from build123d import *

# Parameters (mm, degrees)
CROQUIS1_R              = 2.5
SALIENTE_EXTRUIR1_DEPTH = 60
CORTAR_EXTRUIR1_START   = -10
CORTAR_EXTRUIR1_DEPTH   = 10
CHAFL_N1_SIZE           = 0.2


with BuildPart() as part:
    # Croquis1 → Saliente-Extruir1 (new body)
    with BuildSketch(Plane(origin=(0, 0, 0), x_dir=(1, 0, 0), z_dir=(0, 1, 0))):
        with Locations(Location((0, 0, 0), (0, 0, 270))):
            Circle(CROQUIS1_R)
    extrude(amount=SALIENTE_EXTRUIR1_DEPTH)

    # Croquis2 → Cortar-Extruir1 (cut)
    with BuildSketch(Plane(origin=(0, 60, 0), x_dir=(1, 0, 0), z_dir=(0, 1, 0)).offset(CORTAR_EXTRUIR1_START)):
        with BuildLine():
            Line((-1.5, 2), (1.5, 2))
            ThreePointArc((1.5, 2), (0, 2.5), (-1.5, 2))
        make_face()
    extrude(amount=CORTAR_EXTRUIR1_DEPTH, mode=Mode.SUBTRACT)

    # Chaflán1
    chafl_n1_edges = [part.edges().sort_by_distance(p)[0] for p in [
        (0, 0, -2.5),
        (-2.371708245, 60, 0.790569415),
    ]]
    chamfer(chafl_n1_edges, length=CHAFL_N1_SIZE)


solid = part.part
Design review of the part built by this model. Coordinates are the model's own, in mm. A direction names the side the tool comes from. Round coordinates to 2 decimals unless told otherwise and drop trailing zeros. Write each loop counter-clockwise with the first axis right and the second up, starting at its lowest first coordinate (ties: lowest second). Pieces come first, ordered by that corner, then holes. Notation, with made-up numbers: (70.5, -25) - (122.5, -25) arc R34 cw to (122.5, 5) - close; hole circle Ø11 at (25.25, 28.25). An arc over 180 degrees is marked (long way). Return JSON: item names as keys, results as strings. Group by question number.
Item 1: Machinability: for faces 1 (the face through (0, 55, -2)), 2 (the face through (0, 0, 0)), which of the approach directions +Z, -Z, +X, -X, +Y, -Y give a long, thin tool a straight path to every point of the face, cutting with its end or side? Answer none if there is none.
Item 2: For probe 1 along Z at (x, y) = (-0.1, 9); probe 2 along X at (y, z) = (27.5, -0.2); probe 3 along Z at (x, y) = (-2.15, 34.5), list the stretches that pass through material, from the lowest coordinate up. Write a range as [from, to].
Item 3: Insertion check: P1, Ø1, axis at y = 51, z = 1.5, coming from the +X side; P2, Ø0.5, axis at x = -0.5, z = -2.5, coming from the +Y side; P3, Ø2.5, axis at x = -0.5, y = 52.5, coming from the -Z side. Each pin has a flat end and moves straight along its axis. Give the tip position at first contact, or say it passes through.
Item 4: We need section C-C on y = 29. Write out the cut boundary in (x, z), and give its area (3 significant figures).
Item 5: We need section B-B on y = 54. Write out the cut boundary in (x, z), and give its area (3 significant figures).
Item 6: We need section A-A on x = 0. Write out the cut boundary in (y, z).
Model answer:
{
 "1": {"face 1": "-Z, +X, -X, +Y", "face 2": "+Z, -Z, +X, -X, -Y"},
 "2": {"probe 1": "z = [-2.5, 2.5]", "probe 2": "x = [-2.49, 2.49]", "probe 3": "z = [-1.28, 1.28]"},
 "3": {"P1": "stops at x = 2.29", "P2": "stops at y = 50", "P3": "stops at z = -2"},
 "4": {"outline": "circle Ø5 at (0, 0)", "area": "19.6 mm²"},
 "5": {"outline": "(-1.5, -2) - (1.5, -2) arc R2.5 ccw (long way) to start", "area": "18.6 mm²"},
 "6": {"outline": "(0, -2.3) - (0.2, -2.5) - (50, -2.5) - (50, -2) - (60, -2) - (60, 2.3) - (59.8, 2.5) - (0.2, 2.5) - (0, 2.3) - close"}
}
